from build123d import *

# Parameters (mm, degrees)
SKETCH1_W             = 55
SKETCH1_H             = 22.6
BOSS_EXTRUDE1_DEPTH   = 2
SKETCH2_R             = 8
CUT_EXTRUDE2_DEPTH    = 2
SKETCH2_4_R           = 8
CUT_EXTRUDE3_DEPTH    = 2
SKETCH5_W             = 10
SKETCH5_H             = 4.6
CUT_EXTRUDE4_DEPTH    = 2
SKETCH6_W             = 55
SKETCH6_H             = 2
BOSS_EXTRUDE2_DEPTH   = 18
SKETCH9_W             = 10
SKETCH9_H             = 10
BOSS_EXTRUDE4_DEPTH   = 13
M3X0_5_TAPPED_HOLE1_D = 2.5
M3X0_5_TAPPED_HOLE2_D = 2.5
FILLET1_R             = 5
FILLET2_R             = 5
FILLET4_R             = 1.8
FILLET5_R             = 1.8
CHAMFER2_SIZE         = 1
FILLET10_R            = 1
SKETCH25_R            = 0.75
CUT_EXTRUDE5_DEPTH    = 10


with BuildPart() as part:
    # Sketch1 → Boss-Extrude1 (new body)
    with BuildSketch(Plane.XY):
        with Locations((-1.071942446, 12.368165468)):
            Rectangle(SKETCH1_W, SKETCH1_H)
    extrude(amount=BOSS_EXTRUDE1_DEPTH)

    # Sketch2 → Cut-Extrude2 (cut)
    with BuildSketch(Plane.XY.offset(2)):
        with Locations((-14.371942446, 13.518165468)):
            Circle(SKETCH2_R)
    extrude(amount=-CUT_EXTRUDE2_DEPTH, mode=Mode.SUBTRACT)

    # Sketch2<4> → Cut-Extrude3 (cut)
    with BuildSketch(Plane.XY.offset(2)):
        with Locations((-14.371942446, 13.518165468)):
            Circle(SKETCH2_4_R)
        with Locations((12.228057554, 13.518165468)):
            Circle(SKETCH2_4_R)
    extrude(amount=-CUT_EXTRUDE3_DEPTH, mode=Mode.SUBTRACT)

    # Sketch5 → Cut-Extrude4 (cut)
    with BuildSketch(Plane.XY.offset(2)):
        with Locations((-1.171942446, 21.368165468)):
            Rectangle(SKETCH5_W, SKETCH5_H)
    extrude(amount=-CUT_EXTRUDE4_DEPTH, mode=Mode.SUBTRACT)

    # Sketch6 → Boss-Extrude2 (add)
    with BuildSketch(Plane(origin=(0, 0, 0), x_dir=(-1, 0, 0), z_dir=(0, 0, -1))):
        with Locations((1.071942446, 24.668165468)):
            Rectangle(SKETCH6_W, SKETCH6_H)
    extrude(amount=-BOSS_EXTRUDE2_DEPTH)

    # Sketch9 → Boss-Extrude4 (add)
    with BuildSketch(Plane(origin=(0, 23.668165468, 0), x_dir=(-1, 0, 0), z_dir=(0, -1, 0))):
        with Locations((21.321942446, -10)):
            Rectangle(SKETCH9_W, SKETCH9_H)
        with Locations((-19.178057554, -10)):
            Rectangle(SKETCH9_W, SKETCH9_H)
    extrude(amount=-BOSS_EXTRUDE4_DEPTH)

    # M3x0.5 Tapped Hole1 (through all)
    with Locations(Plane(origin=(0, 23.668165468, 0), x_dir=(-1, 0, 0), z_dir=(0, -1, 0))):
        with Locations((-4.928057554, -10)):
            Hole(M3X0_5_TAPPED_HOLE1_D / 2)

    # M3x0.5 Tapped Hole2 (through all)
    with Locations(Plane(origin=(0, 23.668165468, 0), x_dir=(-1, 0, 0), z_dir=(0, -1, 0))):
        with Locations((7.071942446, -10)):
            Hole(M3X0_5_TAPPED_HOLE2_D / 2)

    # Fillet1
    fillet1_edges = [part.edges().sort_by_distance(p)[0] for p in [
        (-28.571942446, 1.068165468, 1),
    ]]
    fillet(fillet1_edges, radius=FILLET1_R)

    # Fillet2
    fillet2_edges = [part.edges().sort_by_distance(p)[0] for p in [
        (26.428057554, 1.068165468, 1),
    ]]
    fillet(fillet2_edges, radius=FILLET2_R)

    # Fillet4
    fillet4_edges = [part.edges().sort_by_distance(p)[0] for p in [
        (3.828057554, 19.068165468, 1),
    ]]
    fillet(fillet4_edges, radius=FILLET4_R)

    # Fillet5
    fillet5_edges = [part.edges().sort_by_distance(p)[0] for p in [
        (-6.171942446, 19.068165468, 1),
    ]]
    fillet(fillet5_edges, radius=FILLET5_R)

    # Chamfer2
    chamfer2_edges = [part.edges().sort_by_distance(p)[0] for p in [
        (-16.321942446, 36.668165468, 10),
        (-21.321942446, 36.668165468, 5),
        (-26.321942446, 36.668165468, 10),
        (-21.321942446, 36.668165468, 15),
        (24.178057554, 36.668165468, 10),
        (19.178057554, 36.668165468, 5),
        (14.178057554, 36.668165468, 10),
        (19.178057554, 36.668165468, 15),
    ]]
    chamfer(chamfer2_edges, length=CHAMFER2_SIZE)

    # Fillet10
    fillet10_edges = [part.edges().sort_by_distance(p)[0] for p in [
        (26.428057554, 24.668165468, 18),
        (-28.571942446, 24.668165468, 18),
    ]]
    fillet(fillet10_edges, radius=FILLET10_R)

    # Sketch25 → Cut-Extrude5 (cut)
    with BuildSketch(Plane.XY.offset(2)):
        with Locations((20.628057554, 4.268165468)):
            Circle(SKETCH25_R)
        with Locations((20.628057554, 22.768165468)):
            Circle(SKETCH25_R)
        with Locations((-22.871942446, 4.268165468)):
            Circle(SKETCH25_R)
        with Locations((-22.871942446, 22.768165468)):
            Circle(SKETCH25_R)
    extrude(amount=-CUT_EXTRUDE5_DEPTH, mode=Mode.SUBTRACT)


solid = part.part
The listing builds one solid part. Answer for the finished solid, in the listing's coordinates (mm). A direction names the side the tool comes from. Coordinates: 2 decimals unless noted, no trailing zeros. Loops run counter-clockwise (first coordinate to the right, second up) from the corner with the lowest first, then second, coordinate; pieces in that order, holes last.
1) Find section D-D on x = 5.5. Write down the section's boundary in (y, z), then the cut area to 3 significant figures.
2) Flat-ended cylindrical pins translate along their axes: pin 1 Ø1 at (x, z) = (-2, 1) entering from +Y; pin 2 Ø8 at (y, z) = (18, 7) entering from -X; pin 3 Ø3 at (x, z) = (-5, 14.5) entering from -Y; pin 4 Ø10 at (x, y) = (9, 8.5) entering from +Z. Find the tip coordinate at first contact, or state that the pin passes through.
3) Find the intervals of material crossed by L1, parallel to X at y = 24.5, z = 10; L2, parallel to X at y = 29.5, z = 10.25; L3, parallel to Y at x = -2, z = 11.25, in increasing order.
4) Find section A-A on y = 31. Write down the section's boundary in (x, z), then the cut area to 3 significant figures.
5) A tool of negligible diameter and unlimited length cuts with its end or side. For faces 5 (the face through (-1, 13, 2)), 6 (the face through (-16.322, 31, 10)), 7 (the face through (3.828, 22, 1)), 8 (the face through (19, 31, 5)), 9 (the face through (-21, 31, 15)), from which of +Z, -Z, +X, -X, +Y, -Y can it reach the whole face along a straight path? Write none if from no direction.
6) Find section B-B on z = 10. Write down the section's boundary in (x, y), then the cut area to 3 significant figures.
7) Determine the mould class of faces 1 (the face through (19, 36.668, 10)), 2 (the face through (26.428, 19.5, 1.5)), 3 (the face through (-27.146, 2.572, 1.014)), 4 (the face through (14.178, 31, 10)) for opening direction X: pulls with the +X half, pulls with the -X half, needs draft (parallel to the pull), parting line crosses it, or undercut.
8) Find section C-C on x = -13. Write down the section's boundary in (y, z), then the cut area to 3 significant figures.
Values:
1. outline: (1.07, 0) - (9.19, 0) - (9.19, 2) - (1.07, 2) - close; (17.85, 0) - (25.67, 0) - (25.67, 8.89) - (23.67, 8.89) - (23.67, 2) - (17.85, 2) - close; (23.67, 11.11) - (25.67, 11.11) - (25.67, 18) - (23.67, 18) - close
1. area: 59.4 mm2
2. pin 1: stops at y = 25.67
2. pin 2: passes through
2. pin 3: stops at y = 23.67
2. pin 4: stops at z = 2
3. L1: x = -28.57 to -8.32, -5.82 to 3.68, 6.18 to 26.43
3. L2: x = -26.32 to -16.32, 14.18 to 24.18
3. L3: y = 23.67 to 25.67
4. outline: (-26.32, 5) - (-16.32, 5) - (-16.32, 15) - (-26.32, 15) - close; (14.18, 5) - (24.18, 5) - (24.18, 15) - (14.18, 15) - close
4. area: 200 mm2
5. face 5: +Z, +X, -X, -Y
5. face 6: +Z, -Z, +Y
5. face 7: +Z, -Z
5. face 8: -Z, +X, -X, +Y
5. face 9: +Z, +X, -X, +Y
6. outline: (-28.57, 23.67) - (-8.32, 23.67) - (-8.32, 25.67) - (-16.32, 25.67) - (-16.32, 35.67) - (-17.32, 36.67) - (-25.32, 36.67) - (-26.32, 35.67) - (-26.32, 25.67) - (-28.57, 25.67) - close; (-5.82, 23.67) - (3.68, 23.67) - (3.68, 25.67) - (-5.82, 25.67) - close; (6.18, 23.67) - (26.43, 23.67) - (26.43, 25.67) - (24.18, 25.67) - (24.18, 35.67) - (23.18, 36.67) - (15.18, 36.67) - (14.18, 35.67) - (14.18, 25.67) - (6.18, 25.67) - close
6. area: 318 mm2
7. face 1: needs draft
7. face 2: pulls with the +X half
7. face 3: pulls with the -X half
7. face 4: undercut
8. outline: (1.07, 0) - (5.64, 0) - (5.64, 2) - (1.07, 2) - close; (21.4, 0) - (25.67, 0) - (25.67, 18) - (23.67, 18) - (23.67, 2) - (21.4, 2) - close
8. area: 49.7 mm2
